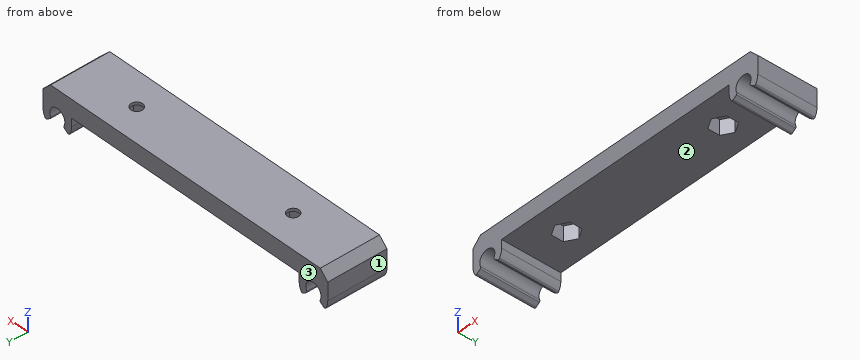
Autodesk Inventor part; units mm, degrees
ref_plane "YZ Plane" through (0, 0, 0) normal (1, 0, 0) x (0, 1, 0)
ref_plane "XZ Plane" through (0, 0, 0) normal (0, 1, 0) x (-1, 0, 0)
ref_plane "XY Plane" through (0, 0, 0) normal (0, 0, 1) x (1, 0, 0)
sketch "Sketch1" plane through (0, 0, 0) normal (0, 1, 0) x (-1, 0, 0)
  line L0 (52.8, -3) -> (-52.8, -3) construction
  line L1 (-52.8, -3) -> (-52.8, 3)
  line L2 (-52.8, 3) -> (52.8, 3) construction
  line L3 (52.8, 3) -> (52.8, -3)
  circle A0 centre (47.5, -5.8) radius 2.8 construction
  circle A1 centre (-47.5, -5.8) radius 2.8 construction
  line L4 (50.3, -5.8) -> (50.3, -3) construction
  line L5 (44.7, -5.8) -> (44.7, -3) construction
  circle A2 centre (47.5, -5.8) radius 5.3 construction
  line L6 (52.8, -5.8) -> (52.8, -3)
  line L7 (42.2, -5.8) -> (42.2, -3)
  arc A3 (51.7589, -8.9546) -> (52.8, -5.8) centre (47.5, -5.8) ccw
  arc A4 (42.2, -5.8) -> (43.2411, -8.9546) centre (47.5, -5.8) ccw
  circle A5 centre (-47.5, -5.8) radius 5.3 construction
  line L8 (0, -3) -> (0, 3) construction
  line L9 (47.5, -5.8) -> (47.5, -3) construction
  line L10 (-47.5, -5.8) -> (-47.5, -3) construction
  line L11 (-42.2, -5.8) -> (-42.2, -3)
  line L12 (-52.8, -5.8) -> (-52.8, -3)
  arc A6 (-43.2411, -8.9546) -> (-42.2, -5.8) centre (-47.5, -5.8) ccw
  arc A7 (-52.8, -5.8) -> (-51.7589, -8.9546) centre (-47.5, -5.8) ccw
  line L13 (42.2, -3) -> (-42.2, -3)
  arc A8 (49.75, -7.4666) -> (45.25, -7.4666) centre (47.5, -5.8) ccw
  line L14 (49.75, -7.4666) -> (51.7589, -8.9546)
  line L15 (45.25, -7.4666) -> (43.2411, -8.9546)
  arc A9 (-45.25, -7.4666) -> (-49.75, -7.4666) centre (-47.5, -5.8) ccw
  line L16 (-45.25, -7.4666) -> (-43.2411, -8.9546)
  line L17 (-49.75, -7.4666) -> (-51.7589, -8.9546)
  line L18 (50, 3) -> (-50, 3)
  line L19 (-50, 3) -> (-52.8, 0.2)
  line L20 (50, 3) -> (52.8, 0.2)
  point P0 (0, 0)
  point P1 (0, 0)
  point P2 (47.5, -3)
  point P3 (-53.25, -3)
  dimension "d0" = 95
  dimension "d1" = 2.5
  dimension "d4" = 6
  dimension "d5" = 6
  dimension "d20" = 5.6
  dimension "d21" = 4.5
  dimension "d22" = 100
extrude "Extrusion1" add sketch "Sketch1" along normal blind 20
fillet "Fillet1" radius 0.5 8 edges at (45.25, 10, -7.4666) (43.2411, 10, -8.9546) (51.7589, 10, -8.9546) (49.75, 10, -7.4666) (-51.7589, 10, -8.9546) (-49.75, 10, -7.4666) (-43.2411, 10, -8.9546) (-45.25, 10, -7.4666)
sketch "Sketch2" plane through (42.2, 0, -3) normal (0, 0, -1) x (-1, 0, 0)
  line L0 (0, 0) -> (84.4, 0) construction
  line L1 (0, 20) -> (84.4, 20) construction
  line L2 (42.2, 20) -> (42.2, 0) construction
  line L3 (13.2, 10) -> (71.2, 10) construction
  line L4 (9.7, 12.0207) -> (13.2, 14.0415)
  line L5 (13.2, 14.0415) -> (16.7, 12.0207)
  line L6 (16.7, 12.0207) -> (16.7, 7.9793)
  line L7 (16.7, 7.9793) -> (13.2, 5.9585)
  line L8 (13.2, 5.9585) -> (9.7, 7.9793)
  line L9 (9.7, 7.9793) -> (9.7, 12.0207)
  line L10 (74.7, 12.0207) -> (74.7, 7.9793)
  line L11 (74.7, 7.9793) -> (71.2, 5.9585)
  line L12 (71.2, 5.9585) -> (67.7, 7.9793)
  line L13 (67.7, 7.9793) -> (67.7, 12.0207)
  line L14 (67.7, 12.0207) -> (71.2, 14.0415)
  line L15 (71.2, 14.0415) -> (74.7, 12.0207)
  point P0 (42.2, 10)
  point P1 (42.2, 10)
  dimension "d9" = 58
  dimension "d10" = 7
extrude "Extrusion2" cut sketch "Sketch2" against normal blind 5
hole "Hole1" at (29, 10, -3) at (-29, 10, -3) direction (0, 0, 1) diameter 3.9 end through all
properties part number "switch_mount"
For this review, take the finished solid that the model builds, in its own axes (mm). Face numbers are marked on the shaded views. Give positions to 0.01 mm unless a question says otherwise; leave off trailing zeros. Loops run counter-clockwise (first coordinate to the right, second up) from the corner with the lowest first, then second, coordinate; pieces in that order, holes last. Notation, with made-up numbers: M 50.5,15.25 L 79.5,15.25 A35 cw 79.5,54.25 Z; hole C 44,6 d1. An arc over 180 degrees is marked long. One line per item, written item: value. Start each with the question number.
Q1. Add section A-A (z = -1.5). Give the boundary of the cut face in (x, y).
Q2. Clearance check with flat-ended pins moving along their axes: pin 1 Ø10 at (x, y) = (9, 7.5) entering from -Z; pin 2 Ø3 at (y, z) = (2.5, -7.5) entering from +X; pin 3 Ø6 at (x, y) = (-29, 10) entering from -Z; pin 4 Ø6.5 at (x, z) = (-47.5, -5.8) entering from -Y. State where each tip first meets the part, or that it passes through.
Q3. For L1, parallel to X at y = 9, z = -5.8; L2, parallel to X at y = 8, z = -3.5; L3, parallel to Y at x = -29, z = 2.55, list the stretches that pass through material, from the lowest coordinate up.
Q4. Add section B-B (x = -34.5). Give the boundary of the cut face in (y, z), and give its area (3 significant figures).
Q5. Add section C-C (y = 2). Give the boundary of the cut face in (x, z), and give its area (3 significant figures).
Q6. Draft analysis for pull direction X (two halves, no side actions). For the marked faces 1, 2 and 3, state which applies: released by +X, released by -X, zero draft, split by the parting line, or undercut.
Q7. Add section D-D (y = 10). Count the separate pieces of the cut face and the enclosed holes in it, and give its area (3 significant figures).
Reply:
1. outline: M -52.8,0 L 52.8,0 L 52.8,20 L -52.8,20 Z; hole M -32.5,7.98 L -29,5.96 L -25.5,7.98 L -25.5,12.02 L -29,14.04 L -32.5,12.02 Z; hole M 25.5,7.98 L 29,5.96 L 32.5,7.98 L 32.5,12.02 L 29,14.04 L 25.5,12.02 Z
2. pin 1: z = -3
2. pin 2: x = 52.8
2. pin 3: z = 2
2. pin 4: y = 0
3. L1: -52.8 to -50.3, -44.7 to -42.2, 42.2 to 44.7, 50.3 to 52.8
3. L2: -52.8 to -49.1, -45.9 to -42.2, 42.2 to 45.9, 49.1 to 52.8
3. L3: 0 to 8.05, 11.95 to 20
4. outline: M 0,-3 L 20,-3 L 20,3 L 0,3 Z
4. area: 120 mm²
5. outline: M -52.8,-5.8 A5.3 ccw -52.06,-8.49 A0.5 ccw -51.34,-8.64 L -50.12,-7.74 A0.5 ccw -49.98,-7.11 A2.8 cw long -45.02,-7.11 A0.5 ccw -44.88,-7.74 L -43.66,-8.64 A0.5 ccw -42.94,-8.49 A5.3 ccw -42.2,-5.8 L -42.2,-3 L 42.2,-3 L 42.2,-5.8 A5.3 ccw 42.94,-8.49 A0.5 ccw 43.66,-8.64 L 44.88,-7.74 A0.5 ccw 45.02,-7.11 A2.8 cw long 49.98,-7.11 A0.5 ccw 50.12,-7.74 L 51.34,-8.64 A0.5 ccw 52.06,-8.49 A5.3 ccw 52.8,-5.8 L 52.8,0.2 L 50,3 L -50,3 L -52.8,0.2 Z
5. area: 686 mm²
6. face 1: released by -X
6. face 2: undercut
6. face 3: zero draft
7. separate pieces: 3
7. enclosed holes: 0
7. area: 608 mm²
